Read the model definition and answer for the solid it produces. Units are mm, in the model's axes. Face numbers are marked on the shaded views. A direction names the side the tool comes from. Coordinates: 2 decimals unless noted, no trailing zeros. Loops run counter-clockwise (first coordinate to the right, second up) from the corner with the lowest first, then second, coordinate; pieces in that order, holes last. Notation, with made-up numbers: M 10,17 L 15,17 A32 cw 15,52 Z; hole C 89.5,50.25 d7. An arc over 180 degrees is marked long. Put each result on its own line as item: value.
from build123d import *

# Parameters (mm, degrees)
SKETCH1_R           = 3.875
SKETCH1_R_2         = 2
BOSS_EXTRUDE1_DEPTH = 0.6
SKETCH2_R           = 3.875
SKETCH2_R_2         = 3.175
BOSS_EXTRUDE2_DEPTH = 2.8
FILLET1_R           = 0.7


with BuildPart() as part:
    # Sketch1 → Boss-Extrude1 (new body)
    with BuildSketch(Plane(origin=(0, 0, 0), x_dir=(0, 1, 0), z_dir=(0, 0, 1))):
        with Locations(Location((0, 0, 0), (0, 0, 270))):
            Circle(SKETCH1_R)
        with Locations(Location((0, 0, 0), (0, 0, 270))):
            Circle(SKETCH1_R_2, mode=Mode.SUBTRACT)
    extrude(amount=BOSS_EXTRUDE1_DEPTH)

    # Sketch2 → Boss-Extrude2 (add)
    with BuildSketch(Plane.XY.offset(0.6)):
        Circle(SKETCH2_R)
        Circle(SKETCH2_R_2, mode=Mode.SUBTRACT)
    extrude(amount=BOSS_EXTRUDE2_DEPTH)

    # Fillet1
    fillet1_edges = [part.edges().sort_by_distance(p)[0] for p in [
        (-3.875, 0, 0),
    ]]
    fillet(fillet1_edges, radius=FILLET1_R)


solid = part.part
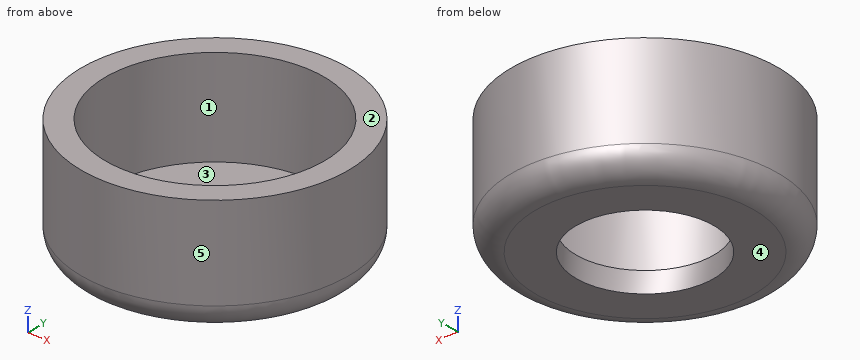
1) Find section A-A, the plane x = 0. Write down the section's boundary in (y, z) (3 decimals), plus the area to 3 significant figures.
Answer list:
outline: M -3.875,0.7 A0.7 ccw -3.175,0 L -2,0 L -2,0.6 L -3.175,0.6 L -3.175,3.4 L -3.875,3.4 Z; M 2,0 L 3.175,0 A0.7 ccw 3.875,0.7 L 3.875,3.4 L 3.175,3.4 L 3.175,0.6 L 2,0.6 Z
area: 5.96 mm^2
2) Find section C-C, the plane z = 1.85. Write down the section's boundary in (x, y) (3 decimals).
Answer list:
outline: C 0,0 d7.75; hole C 0,0 d6.35
3) Which of the six approach directions +Z, -Z, +X, -X, +Y, -Y give full straight-line access (tool end or side, diameter ignored) to the marked faces 1 and 2?
Answer list:
face 1: +Z
face 2: +Z, +X, -X, +Y, -Y
4) Straight lines are drawn through the part: line 1 (Y direction, x = 0, z = 2.5) (3 decimals); line 2 (Z direction, x = -2.25, y = 0.5); line 3 (Y direction, x = 2, z = 2.75). For each, find the intervals that lie inside material, in ascending order. Write a range as [from, to].
Answer list:
line 1: y = [-3.875, -3.175], [3.175, 3.875]
line 2: z = [0, 0.6]
line 3: y = [-3.32, -2.47], [2.47, 3.32]
5) Given pin 1 Ø1 at (y, z) = (2.5, 1.5) entering from +X; pin 2 Ø1.9 at (x, y) = (-1, -1.5) entering from +Z; pin 3 Ø1.5 at (y, z) = (-1, 2.5) entering from +X, each flat-ended and moving along its own axis, determine where each tip first touches the part or whether it passes through.
Answer list:
pin 1: stops at x = 3.32
pin 2: stops at z = 0.6
pin 3: stops at x = 3.87
6) Determine the mould class of the marked faces 3, 4 and 5 for opening direction Y: released by +Y, released by -Y, zero draft, split by the parting line, or undercut.
Answer list:
face 3: undercut
face 4: zero draft
face 5: split by the parting line
